```python
from build123d import *

# Parameters (mm, degrees)
F0_W     = 50
F0_H     = 38
F1_DEPTH = 0.8
F2_W     = 50
F2_H     = 38
F2_W_2   = 23.8
F2_H_2   = 36.4
F3_DEPTH = 43.2
F4_R     = 0.4


with BuildPart() as f1:
    # F0 (on Top) → F1 (new body)
    with BuildSketch(Plane.XY):
        with Locations((-25, 19)):
            Rectangle(F0_W, F0_H)
    extrude(amount=F1_DEPTH)

    # F2 (on face) → F3 (join)
    with BuildSketch(Plane.XY.offset(0.8)):
        with Locations((-25, 19)):
            Rectangle(F2_W, F2_H)
        with Locations((-37.3, 19)):
            Rectangle(F2_W_2, F2_H_2, mode=Mode.SUBTRACT)
        with Locations((-12.7, 19)):
            Rectangle(F2_W_2, F2_H_2, mode=Mode.SUBTRACT)
    extrude(amount=F3_DEPTH)

    # F4
    f4_edges = [f1.edges().sort_by_distance(p)[0] for p in [
        (-50, 0, 22),
        (-49.2, 0.8, 22.4),
        (-49.2, 37.2, 22.4),
        (-50, 38, 22),
        (-25.4, 37.2, 22.4),
        (-25.4, 0.8, 22.4),
    ]]
    fillet(f4_edges, radius=F4_R)


solid = f1.part
```
Work out the finished part from the listing and answer in its coordinate system (mm). A direction names the side the tool comes from. Round coordinates to 2 decimals unless told otherwise and drop trailing zeros. Write each loop counter-clockwise with the first axis right and the second up, starting at its lowest first coordinate (ties: lowest second). Pieces come first, ordered by that corner, then holes. Notation, with made-up numbers: (-40, -7) -> (-13, -7) arc R25 cw to (-13, 23) -> close; hole circle Ø3 at (41, 36). An arc over 180 degrees is marked (long way). Write each question's results on one line, items separated by ' | '.
Q1. Straight lines are drawn through the part: line 1 along X through (y, z) = (36, 27); line 2 along Y through (x, z) = (-33.5, 25); line 3 along Z through (x, y) = (-31, 19). For each, find the intervals that lie inside material, in ascending order. Write a range as [from, to].
Data:
line 1: [-50, -49.2], [-25.4, -24.6], [-0.8, 0] | line 2: [0, 0.8], [37.2, 38] | line 3: [0, 0.8]
Q2. Section B-B, the plane y = 19 is taken. Write down the section's boundary in (x, z).
Data:
outline: (-50, 0) -> (0, 0) -> (0, 44) -> (-0.8, 44) -> (-0.8, 0.8) -> (-24.6, 0.8) -> (-24.6, 44) -> (-25.4, 44) -> (-25.4, 0.8) -> (-49.2, 0.8) -> (-49.2, 44) -> (-50, 44) -> close
Q3. Determine the mould class of faces 1 (the flat face through (-13, 37.2, 22)), 2 (the flat face through (-25, 0, 22)), 3 (the flat face through (-25, 38, 22)), 4 (the flat face through (-25, 19, 0)) for opening direction Y: released by +Y, released by -Y, zero draft, split by the parting line, or undercut.
Data:
face 1: undercut | face 2: released by -Y | face 3: released by +Y | face 4: zero draft
Q4. Section A-A, the plane z = 9.5 is taken. Write down the section's boundary in (x, y), then the cut area to 3 significant figures.
Data:
outline: (-50, 0.4) arc R0.4 ccw to (-49.6, 0) -> (0, 0) -> (0, 38) -> (-49.6, 38) arc R0.4 ccw to (-50, 37.6) -> close; hole (-49.2, 1.2) arc R0.4 ccw to (-48.8, 0.8) -> (-25.8, 0.8) arc R0.4 ccw to (-25.4, 1.2) -> (-25.4, 36.8) arc R0.4 ccw to (-25.8, 37.2) -> (-48.8, 37.2) arc R0.4 ccw to (-49.2, 36.8) -> close; hole (-24.6, 0.8) -> (-0.8, 0.8) -> (-0.8, 37.2) -> (-24.6, 37.2) -> close | area: 167 mm^2
Q5. Section C-C, the plane x = -46.5 is taken. Write down the section's boundary in (y, z).
Data:
outline: (0, 0) -> (38, 0) -> (38, 44) -> (37.2, 44) -> (37.2, 0.8) -> (0.8, 0.8) -> (0.8, 44) -> (0, 44) -> close
Q6. Which of the six approach directions +Z, -Z, +X, -X, +Y, -Y give full straight-line access (tool end or side, diameter ignored) to faces 5 (the flat face through (-50, 19, 22)), 6 (the flat face through (-37, 0.8, 22))?
Data:
face 5: +Z, -Z, -X, +Y, -Y | face 6: +Z
